```python
from build123d import *

# Parameters (mm, degrees)
SKETCH1_R                                      = 9.525
BOSS_EXTRUDE1_DEPTH                            = 9.525
CBORE_FOR_8_SOCKET_HEAD_CAP_SCREW1_D           = 4.4958
CBORE_FOR_8_SOCKET_HEAD_CAP_SCREW1_CBORE_D     = 7.9375
CBORE_FOR_8_SOCKET_HEAD_CAP_SCREW1_CBORE_DEPTH = 4.1656
F_1_16_0_0625_DIAMETER_HOLE1_D                 = 1.5875
F_1_16_0_0625_DIAMETER_HOLE1_DEPTH             = 4.826
F_1_16_0_0625_DIAMETER_HOLE1_TIP               = 0.476933116
F_4_40_TAPPED_HOLE1_D                          = 2.2606
F_4_40_TAPPED_HOLE1_DEPTH                      = 6.35
F_4_40_TAPPED_HOLE1_TIP                        = 0.679152758


with BuildPart() as part:
    # Sketch1 → Boss-Extrude1 (new body)
    with BuildSketch(Plane(origin=(0, 0, 0), x_dir=(1, 0, 0), z_dir=(0, 1, 0))):
        with Locations(Location((0, 0, 0), (0, 0, 90))):
            Circle(SKETCH1_R)
    extrude(amount=BOSS_EXTRUDE1_DEPTH)

    # CBORE for #8 Socket Head Cap Screw1 (through all)
    with Locations(Plane(origin=(0, 9.525, 0), x_dir=(1, 0, 0), z_dir=(0, 1, 0))):
        with Locations((0, 3.175)):
            CounterBoreHole(CBORE_FOR_8_SOCKET_HEAD_CAP_SCREW1_D / 2, CBORE_FOR_8_SOCKET_HEAD_CAP_SCREW1_CBORE_D / 2, CBORE_FOR_8_SOCKET_HEAD_CAP_SCREW1_CBORE_DEPTH)

    # 1/16 (0.0625) Diameter Hole1
    with Locations(Plane(origin=(0, 0, 0.381), x_dir=(0, 0, -1), z_dir=(0, -1, 0))):
        with Locations((0, 0)):
            Hole(F_1_16_0_0625_DIAMETER_HOLE1_D / 2, depth=F_1_16_0_0625_DIAMETER_HOLE1_DEPTH)
            with Locations((0, 0, -(F_1_16_0_0625_DIAMETER_HOLE1_DEPTH + F_1_16_0_0625_DIAMETER_HOLE1_TIP / 2))):  # 118° drill point
                Cone(0, F_1_16_0_0625_DIAMETER_HOLE1_D / 2, F_1_16_0_0625_DIAMETER_HOLE1_TIP, mode=Mode.SUBTRACT)

    # #4-40 Tapped Hole1
    with Locations(Plane(origin=(-6.35, 9.525, 0), x_dir=(0, 0, 1), z_dir=(0, 1, 0))):
        with Locations((0, 0), (0, 12.7), (6.35, 6.35)):
            Hole(F_4_40_TAPPED_HOLE1_D / 2, depth=F_4_40_TAPPED_HOLE1_DEPTH)
            with Locations((0, 0, -(F_4_40_TAPPED_HOLE1_DEPTH + F_4_40_TAPPED_HOLE1_TIP / 2))):  # 118° drill point
                Cone(0, F_4_40_TAPPED_HOLE1_D / 2, F_4_40_TAPPED_HOLE1_TIP, mode=Mode.SUBTRACT)


solid = part.part
```
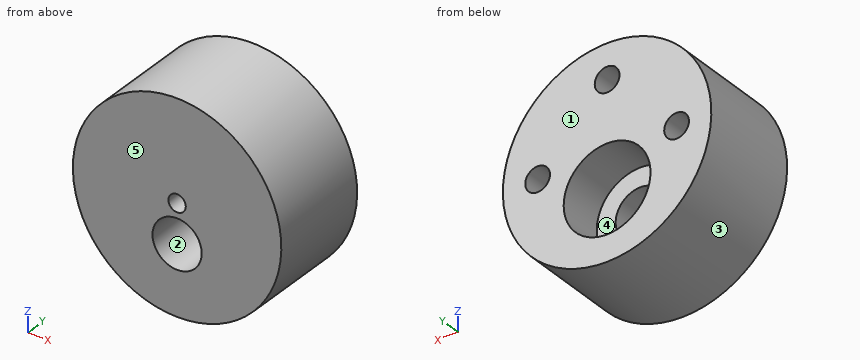
Check sheet for the modelled part. Datum: model origin and axes. Units: mm. Face numbers are marked on the shaded views. A direction names the side the tool comes from. Round coordinates to 2 decimals unless told otherwise and drop trailing zeros. Loops run counter-clockwise (first coordinate to the right, second up) from the corner with the lowest first, then second, coordinate; pieces in that order, holes last. Notation, with made-up numbers: (13, 45.25) - (17, 45.25) arc R22 ccw to (17, 78.25) - close; hole circle Ø3 at (-18.5, 61). An arc over 180 degrees is marked (long way). Answer as a JSON object with one key per item and string values. Group by question number.
Q1. Sectioned sample at A-A, the plane y = 4.5. Count the separate pieces of the cut face and the enclosed holes in it, plus the area to 3 significant figures.
Q2. Set-up check for the marked faces 4 and 5: record each of +Z, -Z, +X, -X, +Y, -Y from which the full face is reachable in a straight line by a thin tool's end or side.
Q3. Gauge pin test, flat ends, axial feed: P1, Ø1.4, axis at x = 0, z = 6.35, coming from the +Y side; P2, Ø2, axis at y = 7, z = 6.5, coming from the -X side; P3, Ø5, axis at x = 0, z = -3.175, coming from the +Y side. Record the tip position at first contact, or that the pin passes through.
Q4. Mould release check, pull along Z, two halves, no side actions. Record for the marked faces 1, 2 and 3: released by +Z, released by -Z, zero draft, split by the parting line, or undercut.
Q5. Sectioned sample at C-C, the plane z = 4.25. Enter the section's corners in (x, y) (3 decimals).
Q6. Scan lines: line 1 along Z through (x, y) = (-0.75, 6); line 2 along X through (y, z) = (3.5, -0.5); line 3 along X through (y, z) = (5, 6.35). Record each from-to range of solid material in increasing order. Write a range as [from, to].
Solution:
{
 "1": {"separate pieces": "1", "enclosed holes": "5", "area": "255 mm²"},
 "2": {"face 4": "+Y", "face 5": "+Z, -Z, +X, -X, -Y"},
 "3": {"P1": "stops at y = 2.92", "P2": "stops at x = -7.78", "P3": "stops at y = 5.36"},
 "4": {"face 1": "zero draft", "face 2": "undercut", "face 3": "split by the parting line"},
 "5": {"outline": "(-8.524, 0) - (8.524, 0) - (8.524, 9.525) - (-8.524, 9.525) - close"},
 "6": {"line 1": "z = [-9.5, -7.07], [0.72, 5.5], [7.2, 9.5]", "line 2": "x = [-9.51, -7.36], [-5.34, 5.34], [7.36, 9.51]", "line 3": "x = [-7.1, -1.13], [1.13, 7.1]"}
}
